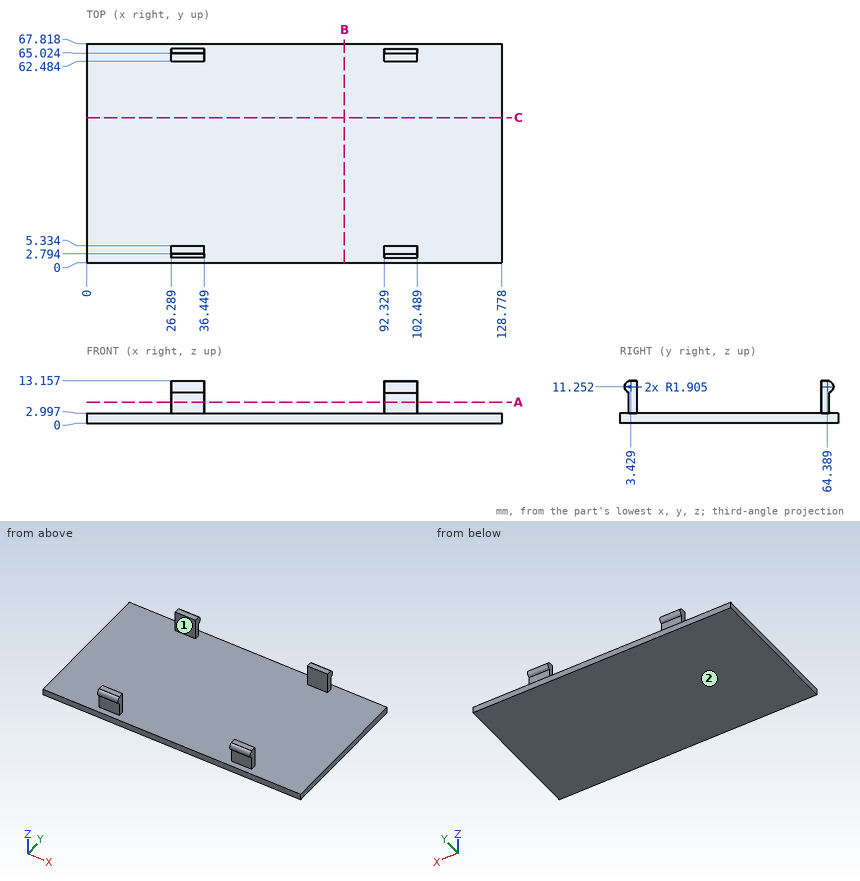
Input: dimensioned drawing with shaded views. Units: mm. Origin: part minimum x, y, z. A direction names the side the tool comes from. Round coordinates to 2 decimals unless told otherwise and drop trailing zeros. Order: outer loops, then holes, each group sorted by start corner. A loop starts at its lowest first (then second) coordinate and runs counter-clockwise, first axis right, second up. Notation, with made-up numbers: (-22, -9.5) -> (-9, -9.5) arc R34 ccw to (-9, 25.5) -> close; hole circle Ø10 at (-2.75, 73). An arc over 180 degrees is marked (long way). Put each result on its own line as item: value. Start each with the question number.
Q1. Section C-C on y = 45. Return the cut outline in (x, z).
Q2. Section B-B on x = 80. Return the cut outline in (y, z), and give its area (3 significant figures).
Q3. Line query: probe 1 along Y at (x, z) = (33.5, 11.25); probe 2 along Z at (x, y) = (51.5, 16); probe 3 along Y at (x, z) = (35, 12). Output: solid intervals per line, ascending.
Q4. Reachability of the marked faces 1 and 2 from +Z, -Z, +X, -X, +Y, -Y: full face, straight path, thin tool, end or side. Return the list, or none.
Q5. Section A-A on z = 6.5. Return the cut outline in (x, y), and give its area (3 significant figures).
Q6. First-contact query: pin 1 (2 mm diameter, centred on y = 49, z = 4.5, fed in from +X); pin 2 (3 mm diameter, centred on x = 32, z = 6, fed in from +Y); pin 3 (1.5 mm diameter, centred on x = 45.5, y = 18.5, fed in from +Z); pin 4 (1.9 mm diameter, centred on y = 3.5, z = 7, fed in from +X). Flat tips, straight axial feed; report the tip coordinate or a pass-through.
Ans:
1. outline: (0, 0) -> (128.78, 0) -> (128.78, 3) -> (0, 3) -> close
2. outline: (0, 0) -> (67.82, 0) -> (67.82, 3) -> (0, 3) -> close
2. area: 203 mm2
3. probe 1: y = 1.52 to 5.33, 62.48 to 66.29
3. probe 2: z = 0 to 3
3. probe 3: y = 1.68 to 5.33, 62.48 to 66.14
4. face 1: +Z, +X, -X
4. face 2: -Z, +X, -X, +Y, -Y
5. outline: (26.29, 2.79) -> (36.45, 2.79) -> (36.45, 5.33) -> (26.29, 5.33) -> close; (26.29, 62.48) -> (36.45, 62.48) -> (36.45, 65.02) -> (26.29, 65.02) -> close; (92.33, 2.79) -> (102.49, 2.79) -> (102.49, 5.33) -> (92.33, 5.33) -> close; (92.33, 62.48) -> (102.49, 62.48) -> (102.49, 65.02) -> (92.33, 65.02) -> close
5. area: 103 mm2
6. pin 1: passes through
6. pin 2: stops at y = 65.02
6. pin 3: stops at z = 3
6. pin 4: stops at x = 102.49
